from build123d import *

# Parameters (mm, degrees)
SKETCH_1_R          = 7.6
SKETCH_1_R_2        = 1.5
EXTRUDE_1_DEPTH     = 3
SKETCH_2_R          = 1
CUT_EXTRUDE_1_DEPTH = 70.858786133
CUT_EXTRUDE_2_DEPTH = 70.858786133
CHAMFER_1_SIZE      = 10
FILLET_2_R          = 2


with BuildPart() as part:
    # 草图1 → 凸台-拉伸1 (new body)
    with BuildSketch(Plane(origin=(0, 0, 0), x_dir=(1, 0, 0), z_dir=(0, 1, 0))):
        with BuildLine():
            Line((-37, 33), (-37, 21))
            Line((-37, 21), (-40, 21))
            Line((-40, 21), (-56.580484914, 9.431183292))
            ThreePointArc((-56.580484914, 9.431183292), (-61.5, 0), (-56.580484914, -9.431183292))
            Line((-56.580484914, -9.431183292), (-40, -21))
            Line((-40, -21), (-37, -21))
            Line((-37, -21), (-37, -33))
            Line((-37, -33), (37, -33))
            Line((37, -33), (37, -21))
            Line((37, -21), (40, -21))
            Line((40, -21), (56.580484914, -9.431183292))
            ThreePointArc((56.580484914, -9.431183292), (61.5, 0), (56.580484914, 9.431183292))
            Line((56.580484914, 9.431183292), (40, 21))
            Line((40, 21), (37, 21))
            Line((37, 21), (37, 33))
            Line((37, 33), (-37, 33))
        make_face()
        with Locations(Location((-50, 0, 0), (0, 0, 270))):
            Circle(SKETCH_1_R, mode=Mode.SUBTRACT)
        with Locations(Location((50, 0, 0), (0, 0, 90))):
            Circle(SKETCH_1_R, mode=Mode.SUBTRACT)
        with Locations(Location((32, 19.25, 0), (0, 0, 90))):
            Circle(SKETCH_1_R_2, mode=Mode.SUBTRACT)
        with Locations(Location((32, -19.25, 0), (0, 0, 90))):
            Circle(SKETCH_1_R_2, mode=Mode.SUBTRACT)
        with Locations(Location((-32, -19.25, 0), (0, 0, 270))):
            Circle(SKETCH_1_R_2, mode=Mode.SUBTRACT)
        with Locations(Location((-32, 19.25, 0), (0, 0, 270))):
            Circle(SKETCH_1_R_2, mode=Mode.SUBTRACT)
        with Locations(Location((-20, 29, 0), (0, 0, 270))):
            Circle(SKETCH_1_R_2, mode=Mode.SUBTRACT)
        with Locations(Location((20, 29, 0), (0, 0, 90))):
            Circle(SKETCH_1_R_2, mode=Mode.SUBTRACT)
    extrude(amount=EXTRUDE_1_DEPTH)

    # 草图2 → 切除-拉伸1 (cut, through all)
    with BuildSketch(Plane(origin=(0, 3, 0), x_dir=(1, 0, 0), z_dir=(0, 1, 0))):
        with Locations((-37, 22)):
            Circle(SKETCH_2_R)
        with Locations((-37, -22)):
            Circle(SKETCH_2_R)
        with Locations((37, -22)):
            Circle(SKETCH_2_R)
        with Locations((37, 22)):
            Circle(SKETCH_2_R)
    extrude(amount=-CUT_EXTRUDE_1_DEPTH, mode=Mode.SUBTRACT)

    # 草图3 → 切除-拉伸2 (cut, through all)
    with BuildSketch(Plane(origin=(0, 3, 0), x_dir=(1, 0, 0), z_dir=(0, 1, 0))):
        Polygon((-27, -26.75), (-27, 25), (27, 25), (27, -26.75), (37, -26.75), (37, -33), (-37, -33), (-37, -26.75), align=None)
    extrude(amount=-CUT_EXTRUDE_2_DEPTH, mode=Mode.SUBTRACT)

    # 倒角1
    chamfer_1_edges = [part.edges().sort_by_distance(p)[0] for p in [
        (-27, 1.5, -25),
        (27, 1.5, -25),
    ]]
    chamfer(chamfer_1_edges, length=CHAMFER_1_SIZE)

    # 圆角2
    fillet_2_edges = [part.edges().sort_by_distance(p)[0] for p in [
        (-27, 1.5, 26.75),
        (27, 1.5, 26.75),
        (-17, 1.5, -25),
        (17, 1.5, -25),
        (27, 1.5, -15),
        (-27, 1.5, -15),
    ]]
    fillet(fillet_2_edges, radius=FILLET_2_R)


solid = part.part
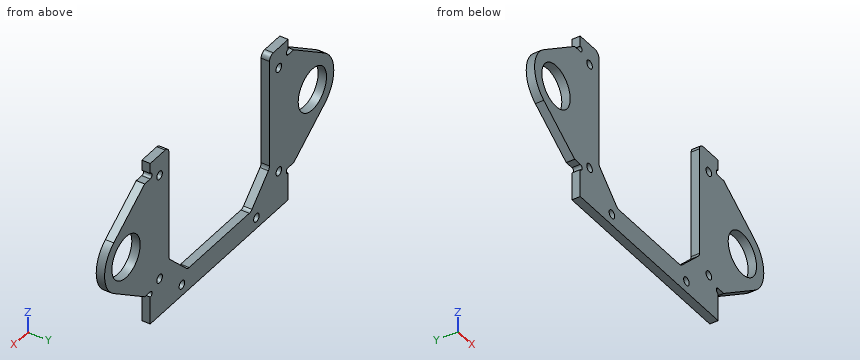
Design review of the part built by this model. Coordinates are the model's own, in mm. Round coordinates to 2 decimals unless told otherwise and drop trailing zeros. Loops run counter-clockwise (first coordinate to the right, second up) from the corner with the lowest first, then second, coordinate; pieces in that order, holes last. Notation, with made-up numbers: M 5,-24.75 L 64,-24.75 A33 ccw 64,14.25 Z; hole C -6.5,30 d7. An arc over 180 degrees is marked long. Answer as a JSON object with one key per item and string values.
Item 1: We need section A-A on z = 0. Give the boundary of the cut face in (x, y), and give its area (3 significant figures).
Answer sheet:
{"outline": "M -61.5,0 L -57.6,0 L -57.6,3 L -61.5,3 Z; M -42.4,0 L -27,0 L -27,3 L -42.4,3 Z; M 27,0 L 42.4,0 L 42.4,3 L 27,3 Z; M 57.6,0 L 61.5,0 L 61.5,3 L 57.6,3 Z", "area": "116 mm^2"}
Item 2: We need section B-B on z = -29. Give the boundary of the cut face in (x, y), and give its area (3 significant figures).
Answer sheet:
{"outline": "M -37,0 L -21.5,0 L -21.5,3 L -37,3 Z; M -18.5,0 L 18.5,0 L 18.5,3 L -18.5,3 Z; M 21.5,0 L 37,0 L 37,3 L 21.5,3 Z", "area": "204 mm^2"}
Item 3: Clearance check with flat-ended pins moving along their axes: P1, Ø9, axis at x = 50, z = 0, coming from the +Y side; P2, Ø1.5, axis at x = -3.5, y = 2, coming from the +Z side; P3, Ø4, axis at x = 32, z = 19.25, coming from the +Y side; P4, Ø0.9, axis at x = 38, y = 1.5, coming from the +Z side. State where each tip first meets the part, or that it passes through.
Answer sheet:
{"P1": "passes through", "P2": "stops at z = -25", "P3": "stops at y = 3", "P4": "stops at z = 21"}
Item 4: We need section C-C on x = 32. Give the boundary of the cut face in (y, z).
Answer sheet:
{"outline": "M 0,-33 L 3,-33 L 3,-20.75 L 0,-20.75 Z; M 0,-17.75 L 3,-17.75 L 3,17.75 L 0,17.75 Z; M 0,20.75 L 3,20.75 L 3,26.75 L 0,26.75 Z"}
Item 5: We need section D-D on y = 0.85. State how many separate pieces and enclosed holes the cut face has, and give its area (3 significant figures).
Answer sheet:
{"separate pieces": "1", "enclosed holes": "8", "area": "2,710 mm^2"}
Item 6: Wall thickness on L1, parallel to X at y = 2.1, z = -29; L2, parallel to X at y = 1.95, z = 0; L3, parallel to X at y = 2.05, z = -19.25: over which ranges is each line inside the solid? List them lowest first. Write a range as from..to.
Answer sheet:
{"L1": "x = -37..-21.5, -18.5..18.5, 21.5..37", "L2": "x = -61.5..-57.6, -42.4..-27, 27..42.4, 57.6..61.5", "L3": "x = -42.51..-33.5, -30.5..-22.75, 22.75..30.5, 33.5..42.51"}
